Verification items for the finished model (mm, model axes). Coordinates: 2 decimals unless noted, no trailing zeros. Order: outer loops, then holes, each group sorted by start corner. A loop starts at its lowest first (then second) coordinate and runs counter-clockwise, first axis right, second up.
Q1. Depth check by flat-ended pin: P1, Ø5.5, axis at x = 0, z = 40.64, coming from the +Y side; P2, Ø1.5, axis at x = 31.5, y = -1.5, coming from the +Z side. Enter the tip coordinate at first touch or a pass-through.
Q2. Thickness scan on line 1 (Z direction, x = 0, y = -3.1); line 2 (Z direction, x = 40.64, y = -1.1); line 3 (Z direction, x = -59, y = -1.15). Record the ranges inside material, lowest first.
Q3. Cross-section at B-B, the plane x = 0. Record the boundary of the cut face in (y, z).
Q4. Cross-section at C-C, the plane x = 40.64. Record the boundary of the cut face in (y, z), and give its area (3 significant figures).
Q5. Cross-section at D-D, the plane y = -3.35. Record the boundary of the cut face in (x, z).
Q6. Cross-section at A-A, the plane z = 0. Record the boundary of the cut face in (x, y), and give its area (3 significant figures).
from build123d import *

# Parameters (mm, degrees)
F0_W        = 129.54
F0_H        = 129.54
F0_R        = 3.39979
F1_DEPTH    = 3.9878
F2_T1_DEPTH = 154.3459968354
F2_T3_DEPTH = 154.3459968354


# Not quite as in the source:
# - a fillet or chamfer that OpenCascade refuses, or shapes differently, is made with other operations: its cross-section is extruded or revolved along the edge and cut away or added


with BuildPart() as f1:
    # F0 (on Front) → F1 (new body)
    with BuildSketch(Plane.XZ):
        Rectangle(F0_W, F0_H)
        with Locations((0, -40.64)):
            Circle(F0_R, mode=Mode.SUBTRACT)
        with Locations((-40.64, 0)):
            Circle(F0_R, mode=Mode.SUBTRACT)
        Circle(F0_R, mode=Mode.SUBTRACT)
        with Locations((40.64, 0)):
            Circle(F0_R, mode=Mode.SUBTRACT)
        with Locations((0, 40.64)):
            Circle(F0_R, mode=Mode.SUBTRACT)
    extrude(amount=F1_DEPTH)

    # F2: fillet of radius 5.08 on 4 edges, made by hand

    # F2_s2 → F2_t1 (cut)
    with BuildSketch(Plane.XY.offset(-77.1729984177)):
        with BuildLine():
            ThreePointArc((-64.77, -3.9878), (-62.9914115108, -1.1205318539), (-59.8088006329, 0))
            Line((-59.8088006329, 0), (-64.77, 0))
            Line((-64.77, 0), (-64.77, -3.9878))
        make_face()
        with BuildLine():
            ThreePointArc((64.77, -3.9878), (62.9914115108, -1.1205318539), (59.8088006329, 0))
            Line((59.8088006329, 0), (64.77, 0))
            Line((64.77, 0), (64.77, -3.9878))
        make_face()
    extrude(amount=F2_T1_DEPTH, mode=Mode.SUBTRACT)

    # F2_s4 → F2_t3 (cut)
    with BuildSketch(Plane.YZ.offset(-77.1729984177)):
        with BuildLine():
            ThreePointArc((-3.9878, -64.77), (-1.1205318539, -62.9914115108), (0, -59.8088006329))
            Line((0, -59.8088006329), (0, -64.77))
            Line((0, -64.77), (-3.9878, -64.77))
        make_face()
        with BuildLine():
            ThreePointArc((-3.9878, 64.77), (-1.1205318539, 62.9914115108), (0, 59.8088006329))
            Line((0, 59.8088006329), (0, 64.77))
            Line((0, 64.77), (-3.9878, 64.77))
        make_face()
    extrude(amount=F2_T3_DEPTH, mode=Mode.SUBTRACT)


solid = f1.part
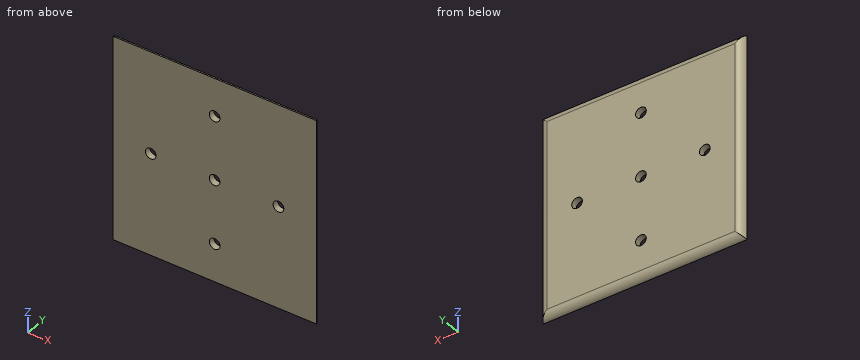
Check values:
1. P1: passes through
1. P2: stops at z = 64.03
2. line 1: z = -64.49 to -44.04, -37.24 to -3.4, 3.4 to 37.24, 44.04 to 64.49
2. line 2: z = -62.97 to -3.4, 3.4 to 62.97
2. line 3: z = -63.03 to 63.03
3. outline: (-3.99, -64.77) arc R5.08 ccw to (0, -59.81) - (0, -44.04) - (-3.99, -44.04) - close; (-3.99, -37.24) - (0, -37.24) - (0, -3.4) - (-3.99, -3.4) - close; (-3.99, 3.4) - (0, 3.4) - (0, 37.24) - (-3.99, 37.24) - close; (-3.99, 44.04) - (0, 44.04) - (0, 59.81) arc R5.08 ccw to (-3.99, 64.77) - close
4. outline: (-3.99, -64.77) arc R5.08 ccw to (0, -59.81) - (0, -3.4) - (-3.99, -3.4) - close; (-3.99, 3.4) - (0, 3.4) - (0, 59.81) arc R5.08 ccw to (-3.99, 64.77) - close
4. area: 479 mm2
5. outline: (-64.59, -64.59) - (64.59, -64.59) - (64.59, 64.59) - (-64.59, 64.59) - close; hole circle Ø6.8 at (-40.64, 0); hole circle Ø6.8 at (0, -40.64); hole circle Ø6.8 at (0, 0); hole circle Ø6.8 at (0, 40.64); hole circle Ø6.8 at (40.64, 0)
6. outline: (-64.77, -3.99) - (-44.04, -3.99) - (-44.04, 0) - (-59.81, 0) arc R5.08 ccw to start; (-37.24, -3.99) - (-3.4, -3.99) - (-3.4, 0) - (-37.24, 0) - close; (3.4, -3.99) - (37.24, -3.99) - (37.24, 0) - (3.4, 0) - close; (44.04, -3.99) - (64.77, -3.99) arc R5.08 ccw to (59.81, 0) - (44.04, 0) - close
6. area: 425 mm2
